Verification items for the finished model (mm, model axes). A direction names the side the tool comes from. Round coordinates to 2 decimals unless told otherwise and drop trailing zeros. Write each loop counter-clockwise with the first axis right and the second up, starting at its lowest first coordinate (ties: lowest second). Pieces come first, ordered by that corner, then holes. Notation, with made-up numbers: (-7.5, 84) - (5.5, 84) arc R20 cw to (5.5, 106) - close; hole circle Ø5 at (2.5, 34). An arc over 180 degrees is marked (long way). Write each question's results on one line, items separated by ' | '.
Autodesk Inventor part; units mm, degrees
ref_plane "Work Plane1" through (0, 0, -61.468) normal (0, 0, -1) x (-1, 0, 0)
ref_plane "Work Plane2" through (31.467332, -7.777429, -126.238) normal (0, 0, -1) x (-1, 0, 0)
ref_plane "YZ Plane" through (0, 0, 0) normal (1, 0, 0) x (0, 1, 0)
sketch "Sketch1" plane through (0, 0, 0) normal (0, 0, 1) x (1, 0, 0)
  line L0 (-20.399473, 8.732571) -> (20.240527, 8.732571)
  line L1 (20.240527, 8.732571) -> (20.240527, -7.777429)
  line L2 (20.240527, -7.777429) -> (-20.399473, -7.777429)
  line L3 (-20.399473, -7.777429) -> (-20.399473, 8.732571)
  point P0 (0, 0)
  dimension "d0" = 40.64
  dimension "d1" = 16.51
extrude "Extrusion1" add sketch "Sketch1" against normal blind 27.178
sketch "Sketch2" plane through (0, 0, 0) normal (0, 0, 1) x (1, 0, 0)
  line L0 (20.240527, -7.777429) -> (-20.399473, -7.777429)
  line L1 (-20.399473, -7.777429) -> (-20.399473, -5.491429)
  line L2 (-20.399473, -7.777429) -> (-20.399473, 8.732571)
  line L3 (-20.399473, -5.491429) -> (-15.065473, -5.491429)
  line L4 (-15.065473, -5.491429) -> (-15.065473, -5.745429)
  line L5 (20.240527, -7.777429) -> (20.240527, -5.491429)
  line L6 (20.240527, 8.732571) -> (20.240527, -7.777429)
  line L7 (20.240527, -5.491429) -> (14.906527, -5.491429)
  line L8 (14.906527, -5.491429) -> (14.906527, -5.745429)
  line L9 (-15.065473, -5.745429) -> (14.906527, -5.745429)
  point P0 (0, 0)
  dimension "d4" = 2.286
  dimension "d5" = 5.334
  dimension "d6" = 0.254
  dimension "d7" = 2.286
  dimension "d8" = 5.334
  dimension "d9" = 0.254
extrude "Extrusion2" add sketch "Sketch2" along normal blind 2.032
sketch "Sketch3" plane through (0, 0, 0) normal (0, 0, 1) x (1, 0, 0)
  line L0 (-20.399473, 8.732571) -> (-20.399473, -5.491429)
  line L1 (20.240527, 8.732571) -> (-20.399473, 8.732571)
  line L2 (14.906527, -5.745429) -> (-15.065473, -5.745429)
  line L3 (-15.065473, 8.732571) -> (-15.065473, -5.745429)
  line L4 (-15.065473, -5.745429) -> (14.906527, -5.745429)
  line L5 (14.906527, -5.745429) -> (14.906527, 8.732571)
  line L6 (-15.065473, 8.732571) -> (14.906527, 8.732571)
  point P0 (0, 0)
  dimension "d12" = 5.334
extrude "Extrusion3" cut sketch "Sketch3" against normal blind 26.416
ref_plane "Work Plane1" through (0, 0, -61.468) normal (0, 0, -1) x (-1, 0, 0)
sketch "Sketch6" plane through (0, 0, -27.178) normal (0, 0, -1) x (-1, 0, 0)
  line L0 (20.399473, -7.777429) -> (-20.240527, -7.777429)
  point P0 (0, 0)
sketch "Sketch8" plane through (0, 0, -61.468) normal (0, 0, -1) x (-1, 0, 0)
  line L0 (0, 12.542354) -> (44.128566, 12.542354)
  line L1 (-20.240527, -7.777429) -> (20.399473, -7.777429)
  line L2 (0.079473, -7.777429) -> (44.128566, -7.777429)
  line L3 (-31.467332, 12.542354) -> (48.234468, 12.542354)
  line L4 (48.234468, 12.542354) -> (48.234468, -7.777429)
  line L5 (48.234468, -7.777429) -> (-31.467332, -7.777429)
  line L6 (-31.467332, -7.777429) -> (-31.467332, 12.542354)
  line L7 (-31.467332, 12.542354) -> (48.234468, 12.542354)
  line L8 (48.234468, 12.542354) -> (48.234468, -7.777429)
  line L9 (48.234468, -7.777429) -> (-31.467332, -7.777429)
  line L10 (-31.467332, -7.777429) -> (-31.467332, 12.542354)
  point P0 (0, 0)
sketch "Sketch8 outline for Loft1" plane through (0, 0, -61.468) normal (0, 0, -1) x (-1, 0, 0)
  line L0 (48.234468, 12.542354) -> (-31.467332, 12.542354)
  line L1 (48.234468, -7.777429) -> (48.234468, 12.542354)
  line L2 (-31.467332, -7.777429) -> (48.234468, -7.777429)
  line L3 (-31.467332, 12.542354) -> (-31.467332, -7.777429)
loft "Loft1" add profiles "Sketch8 outline for Loft1" section 1 edges at (-0.079473, -7.777429, -27.178) (-20.399473, 0.477571, -27.178) (-0.079473, 8.732571, -27.178) (20.240527, 0.477571, -27.178)
ref_plane "Work Plane2" through (31.467332, -7.777429, -126.238) normal (0, 0, -1) x (-1, 0, 0)
extrude "Extrusion4" add sketch "Sketch8" along normal blind 64.77
sketch "Sketch9" plane through (0, 0, -126.238) normal (0, 0, -1) x (-1, 0, 0)
  line L0 (40.614468, -7.777429) -> (40.614468, 12.542354)
  line L1 (-31.467332, 12.542354) -> (48.234468, 12.542354)
  line L2 (40.614468, 12.542354) -> (-21.615532, 12.542354)
  line L3 (-21.615532, 12.542354) -> (-21.615532, -7.777429)
  line L4 (-20.240527, -7.777429) -> (-31.467332, -7.777429)
  line L5 (-21.615532, -7.777429) -> (40.614468, -7.777429)
  point P0 (0, 0)
  point P1 (48.234468, -7.777429)
  dimension "d27" = 7.62
  dimension "d28" = 62.23
extrude "Extrusion5" cut sketch "Sketch9" against normal blind 39.37
sketch "Sketch10" plane through (21.615532, -7.777429, -126.238) normal (-1, 0, 0) x (0, 0, 1)
  point P0 (126.238, 7.777429)
sketch "Sketch11" plane through (31.467332, -7.777429, -61.468) normal (1, 0, 0) x (0, 0, -1)
  line L0 (64.77, 0) -> (64.77, 20.319783)
  line L1 (64.77, 10.159891) -> (54.356, 10.159891)
  circle A0 centre (54.356, 10.159891) radius 2.54
  circle A1 centre (54.356, 10.159891) radius 4.064
  point P0 (-61.468, 7.777429)
  dimension "d31" = 10.414
  dimension "d32" = 5.08
  dimension "d33" = 8.128
extrude "Extrusion6" cut sketch "Sketch11" against normal through all contours A0
sketch "Sketch12" plane through (-20.399473, -5.491429, 0) normal (-1, 0, 0) x (0, 0, 1)
  line L0 (-27.178, -2.286) -> (2.032, -2.286)
  line L1 (-20.32, -2.286) -> (-15.24, -2.286) construction
  line L2 (-20.32, 2.794) -> (-15.24, 2.794)
  line L3 (-15.24, 2.794) -> (-15.24, 14.224)
  line L4 (-20.32, 2.794) -> (-20.32, 14.224)
  line L5 (-20.32, 14.224) -> (-15.24, 14.224)
  point P0 (0, 5.491429)
  point P1 (-27.178, 14.224)
  dimension "d36" = 6.858
  dimension "d37" = 5.08
  dimension "d39" = 5.08
extrude "Extrusion7" cut sketch "Sketch12" against normal blind 25.4
sketch "Sketch13" plane through (0, 0, 0) normal (0, 0, 1) x (1, 0, 0)
  line L0 (-15.065473, -5.491429) -> (-20.399473, -5.491429)
  line L1 (-20.399473, -5.491429) -> (-17.605473, -5.491429)
  circle A0 centre (-17.605473, 2.890571) radius 1.27
  line L2 (20.240527, -5.491429) -> (14.906527, -5.491429)
  line L3 (20.240527, -5.491429) -> (17.446527, -5.491429)
  circle A1 centre (17.446527, 2.890571) radius 1.27
  point P0 (0, 0)
  dimension "d42" = 2.794
  dimension "d44" = 2.54
  dimension "d45" = 2.794
  dimension "d47" = 2.54
extrude "Extrusion8" cut sketch "Sketch13" against normal blind 2.54
sketch "Sketch15" plane through (31.467332, -7.777429, -61.468) normal (1, 0, 0) x (0, 0, -1)
  circle A0 centre (54.356, 10.159891) radius 2.54
  circle A1 centre (54.356, 10.159891) radius 4.064
  point P0 (-61.468, 7.777429)
  dimension "d51" = 8.128
extrude "Extrusion9" cut sketch "Sketch15" against normal blind 3.81 contours A0 | A1
sketch "Sketch16" plane through (21.615532, -7.777429, -126.238) normal (-1, 0, 0) x (0, 0, 1)
  point P0 (126.238, 7.777429)
sketch "Sketch17" plane through (21.615532, -7.777429, -126.238) normal (-1, 0, 0) x (0, 0, 1)
  circle A0 centre (10.414, 10.159891) radius 2.54
  circle A1 centre (10.414, 10.159891) radius 4.064
  point P0 (126.238, 7.777429)
  dimension "d54" = 8.128
extrude "Extrusion10" cut sketch "Sketch17" against normal blind 3.81 contours A0 | A1
sketch "Sketch18" plane through (-40.614468, -7.777429, -126.238) normal (1, 0, 0) x (0, 0, -1)
  circle A0 centre (-10.414, 10.159891) radius 2.54
  line L0 (-8.246516, 6.425305) -> (-12.564505, 6.415502)
  line L1 (-12.564505, 6.415502) -> (-14.731989, 10.150089)
  line L2 (-14.731989, 10.150089) -> (-12.581484, 13.894478)
  line L3 (-12.581484, 13.894478) -> (-8.263495, 13.904281)
  line L4 (-8.263495, 13.904281) -> (-6.096011, 10.169694)
  line L5 (-6.096011, 10.169694) -> (-8.246516, 6.425305)
  point P0 (-126.238, 7.777429)
extrude "Extrusion12" cut sketch "Sketch18" against normal blind 3.81
equation "\"d48\" = d47"
(1) Go/stop test with flat-tipped pins: pin 1 Ø3.5 at (x, y) = (-17.61, 2.89) entering from +Z; pin 2 Ø5.5 at (x, z) = (-18, -18) entering from +Y; pin 3 Ø8 at (x, y) = (-4.5, 10) entering from -Z. Record where each tip stops, or that it passes through.
Answer:
pin 1: z = 0 | pin 2: y = 8.73 | pin 3: z = -86.87
(2) Section check A-A (z = -106.5). Record the cut outline in (x, y).
Answer:
outline: (-48.23, -7.78) - (-40.61, -7.78) - (-40.61, 12.54) - (-48.23, 12.54) - close; (21.62, -7.78) - (31.47, -7.78) - (31.47, 12.54) - (21.62, 12.54) - close
(3) Thickness scan on L1, parallel to X at y = 6.5, z = -24.5; L2, parallel to X at y = 5, z = -89; L3, parallel to Z at x = 8, y = 6.5. Record the ranges inside material, lowest first.
Answer:
L1: -20.4 to -15.07, 14.91 to 20.24 | L2: -48.23 to -40.61, 21.62 to 31.47 | L3: -86.87 to -26.42
(4) Mould release check, pull along Z, two halves, no side actions. Record for faces 1 (the flat face through (20.241, 1, -12)), 2 (the flat face through (-18, 3, -2.54)), 3 (the flat face through (-42.49, 4.29, -119.04)): released by +Z, released by -Z, zero draft, split by the parting line, or undercut.
Answer:
face 1: zero draft | face 2: released by +Z | face 3: undercut
(5) Section check B-B (z = -18). Record the cut outline in (x, y), plus the area to 3 significant figures.
Answer:
outline: (-20.4, -7.78) - (20.24, -7.78) - (20.24, 8.73) - (14.91, 8.73) - (14.91, -5.75) - (-15.07, -5.75) - (-15.07, -2.7) - (-20.4, -2.7) - close | area: 176 mm2
(6) Set-up check for faces 4 (the flat face through (0, 2, -26.416)), 5 (the flat face through (-40.614, 2, -107)), 6 (the cylindrical face through (-16.394, 3.272, -1.252)), 7 (the cylindrical face through (23.494, 3.603, -111.948)), 8 (the flat face through (19, 2, 0)): record each of +Z, -Z, +X, -X, +Y, -Y from which the full face is reachable in a straight line by a thin tool's end or side.
Answer:
face 4: +Z, +Y | face 5: -Z, +Y, -Y | face 6: +Z | face 7: none | face 8: +Z, +X, -X, +Y
